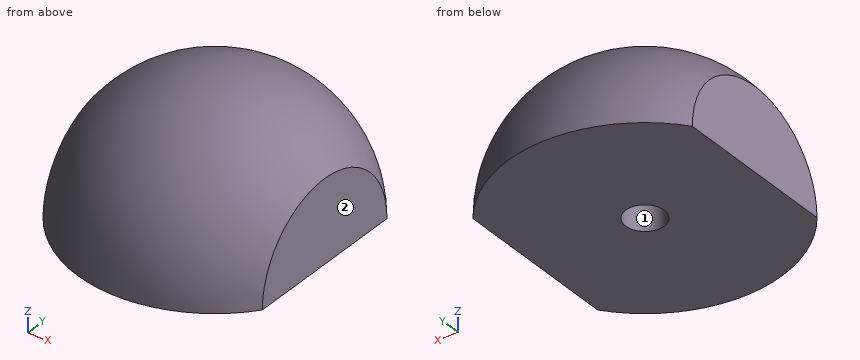
from build123d import *

# Parameters (mm, degrees)
REVOLVE1_ANGLE     = 180
SKETCH3_W          = 56.622410577
SKETCH3_H          = 52.672009839
SKETCH3_W_2        = 24
SKETCH3_H_2        = 38.977287281
CUT_EXTRUDE1_DEPTH = 10
SKETCH4_R          = 2.1
CUT_EXTRUDE2_DEPTH = 8


with BuildPart() as part:
    # Sketch2 → Revolve1 (revolve)
    with BuildSketch(Plane.XY):
        with BuildLine():
            Line((0, 0), (0, 30))
            ThreePointArc((0, 30), (-15, 15), (0, 0))
        make_face()
    revolve(axis=Axis((0, 0, 0), (0, 1, 0)), revolution_arc=REVOLVE1_ANGLE)

    # Sketch3 → Cut-Extrude1 (cut)
    with BuildSketch(Plane(origin=(0, 0, 0), x_dir=(-1, 0, 0), z_dir=(0, 0, -1))):
        with Locations((-0.219466708, 13.463733046)):
            Rectangle(SKETCH3_W, SKETCH3_H)
        with Locations((0, 15.219466708)):
            Rectangle(SKETCH3_W_2, SKETCH3_H_2, mode=Mode.SUBTRACT)
    extrude(amount=-CUT_EXTRUDE1_DEPTH, mode=Mode.SUBTRACT)

    # Sketch4 → Cut-Extrude2 (cut)
    with BuildSketch(Plane(origin=(0, 0, 0), x_dir=(-1, 0, 0), z_dir=(0, 0, -1))):
        with Locations((0, 15)):
            Circle(SKETCH4_R)
    extrude(amount=-CUT_EXTRUDE2_DEPTH, mode=Mode.SUBTRACT)


solid = part.part
Verification items for the finished model (mm, model axes). Face numbers are marked on the shaded views. Round coordinates to 2 decimals unless told otherwise and drop trailing zeros. Order: outer loops, then holes, each group sorted by start corner. A loop starts at its lowest first (then second) coordinate and runs counter-clockwise, first axis right, second up. Notation, with made-up numbers: (86, -12) -> (96, -12) arc R16 ccw to (96, -4) -> close; hole circle Ø10 at (59, -27.5). An arc over 180 degrees is marked (long way). Put each result on its own line as item: value.
1) Section check C-C (x = 0). Record the cut outline in (y, z).
Final values:
outline: (0, 0) -> (12.9, 0) -> (12.9, 8) -> (17.1, 8) -> (17.1, 0) -> (30, 0) arc R15 ccw to start
2) Section check D-D (z = 13.25). Record the cut outline in (x, y), then the cut area to 3 significant figures.
Final values:
outline: circle Ø14.06 at (0, 15)
area: 155 mm^2
3) Section check A-A (y = 15). Record the cut outline in (x, z), then the cut area to 3 significant figures.
Final values:
outline: (-12, 0) -> (-2.1, 0) -> (-2.1, 8) -> (2.1, 8) -> (2.1, 0) -> (12, 0) -> (12, 9) arc R15 ccw to (-12, 9) -> close
area: 283 mm^2
4) Section check B-B (z = 6.25). Record the cut outline in (x, y).
Final values:
outline: (-12, 8.52) arc R13.64 ccw to (12, 8.52) -> (12, 21.48) arc R13.64 ccw to (-12, 21.48) -> close; hole circle Ø4.2 at (0, 15)
5) Depth check by flat-ended pin: pin 1 (2 mm diameter, centred on x = -8, z = 10, fed in from +Y); pin 2 (2.5 mm diameter, centred on x = 0, y = 15, fed in from +Z); pin 3 (1.3 mm diameter, centred on x = -0.5, y = 15.5, fed in from -Z). Enter the tip coordinate at first touch or a pass-through.
Final values:
pin 1: stops at y = 24.25
pin 2: stops at z = 15
pin 3: stops at z = 8
6) Mould release check, pull along Y, two halves, no side actions. Record for the marked faces 1 and 2: +Y half, -Y half, draft (parallel to the pull), parting line (faces both ways), or undercut.
Final values:
face 1: undercut
face 2: draft
7) Material ranges on line 1 (Z direction, x = -9, y = 13.75); line 2 (Y direction, x = 0.5, z = 12); line 3 (Y direction, x = 0, z = 3.5), recorded low to high.
Final values:
line 1: z = 0 to 11.93
line 2: y = 6.01 to 23.99
line 3: y = 0.41 to 12.9, 17.1 to 29.59
